from build123d import *

# Parameters (mm, degrees)
SKETCH1_W           = 10
SKETCH1_H           = 90
BOSS_EXTRUDE1_DEPTH = 10
CUT_EXTRUDE1_DEPTH  = 91
CUT_EXTRUDE2_DEPTH  = 91
CUT_EXTRUDE3_DEPTH  = 91
CUT_EXTRUDE4_DEPTH  = 91
FILLET1_R           = 0.2


with BuildPart() as part:
    # Sketch1 → Boss-Extrude1 (new body)
    with BuildSketch(Plane(origin=(0, 5, 0), x_dir=(1, 0, 0), z_dir=(0, 1, 0))):
        Rectangle(SKETCH1_W, SKETCH1_H)
    extrude(amount=-BOSS_EXTRUDE1_DEPTH)

    # Sketch2 → Cut-Extrude1 (cut, through all)
    with BuildSketch(Plane.XY.offset(45)):
        with BuildLine():
            Line((5, 1.5), (4, 1.5))
            Line((4, 1.5), (4, 2.759344808))
            ThreePointArc((4, 2.759344808), (3.870199868, 2.946619949), (3.649280215, 2.890811711))
            Line((3.649280215, 2.890811711), (2, 1))
            Line((2, 1), (2, -1))
            Line((2, -1), (3.649280215, -2.890811711))
            ThreePointArc((3.649280215, -2.890811711), (3.870199868, -2.946619949), (4, -2.759344808))
            Line((4, -2.759344808), (4, -1.5))
            Line((4, -1.5), (5, -1.5))
            Line((5, -1.5), (5, 1.5))
        make_face()
    extrude(amount=-CUT_EXTRUDE1_DEPTH, mode=Mode.SUBTRACT)

    # Sketch3 → Cut-Extrude2 (cut, through all)
    with BuildSketch(Plane.XY.offset(45)):
        with BuildLine():
            Line((1.5, -5), (1.5, -4))
            Line((1.5, -4), (2.759344808, -4))
            ThreePointArc((2.759344808, -4), (2.946619949, -3.870199868), (2.890811711, -3.649280215))
            Line((2.890811711, -3.649280215), (1, -2))
            Line((1, -2), (-1, -2))
            Line((-1, -2), (-2.890811711, -3.649280215))
            ThreePointArc((-2.890811711, -3.649280215), (-2.946619949, -3.870199868), (-2.759344808, -4))
            Line((-2.759344808, -4), (-1.5, -4))
            Line((-1.5, -4), (-1.5, -5))
            Line((-1.5, -5), (1.5, -5))
        make_face()
    extrude(amount=-CUT_EXTRUDE2_DEPTH, mode=Mode.SUBTRACT)

    # Sketch4 → Cut-Extrude3 (cut, through all)
    with BuildSketch(Plane.XY.offset(45)):
        with BuildLine():
            Line((-5, -1.5), (-4, -1.5))
            Line((-4, -1.5), (-4, -2.759344808))
            ThreePointArc((-4, -2.759344808), (-3.870199868, -2.946619949), (-3.649280215, -2.890811711))
            Line((-3.649280215, -2.890811711), (-2, -1))
            Line((-2, -1), (-2, 1))
            Line((-2, 1), (-3.649280215, 2.890811711))
            ThreePointArc((-3.649280215, 2.890811711), (-3.870199868, 2.946619949), (-4, 2.759344808))
            Line((-4, 2.759344808), (-4, 1.5))
            Line((-4, 1.5), (-5, 1.5))
            Line((-5, 1.5), (-5, -1.5))
        make_face()
    extrude(amount=-CUT_EXTRUDE3_DEPTH, mode=Mode.SUBTRACT)

    # Sketch5 → Cut-Extrude4 (cut, through all)
    with BuildSketch(Plane.XY.offset(45)):
        with BuildLine():
            Line((-1.5, 5), (-1.5, 4))
            Line((-1.5, 4), (-2.759344808, 4))
            ThreePointArc((-2.759344808, 4), (-2.946619949, 3.870199868), (-2.890811711, 3.649280215))
            Line((-2.890811711, 3.649280215), (-1, 2))
            Line((-1, 2), (1, 2))
            Line((1, 2), (2.890811711, 3.649280215))
            ThreePointArc((2.890811711, 3.649280215), (2.946619949, 3.870199868), (2.759344808, 4))
            Line((2.759344808, 4), (1.5, 4))
            Line((1.5, 4), (1.5, 5))
            Line((1.5, 5), (-1.5, 5))
        make_face()
    extrude(amount=-CUT_EXTRUDE4_DEPTH, mode=Mode.SUBTRACT)

    # Sketch6 → Cut-Revolve1 (revolve, cut)
    with BuildSketch(Plane(origin=(0, 0, 0), x_dir=(1, 0, 0), z_dir=(0, 1, 0))):
        Polygon((1.499999999, 37), (1.25, 36.849784845), (1.25, -36.849784845), (1.499999999, -37), (1.499999999, -45), (0, -45), (0, 45), (1.499999999, 45), align=None)
    revolve(axis=Axis((0, 0, -45), (0, 0, 1)), mode=Mode.SUBTRACT)

    # Fillet1
    fillet1_edges = [part.edges().sort_by_distance(p)[0] for p in [
        (-5, -5, 0),
        (-1.5, 5, 0),
        (1.5, 5, 0),
        (1.5, 4, 0),
        (1, 2, 0),
        (-1, 2, 0),
        (-1.5, 4, 0),
        (5, 1.5, 0),
        (5, -1.5, 0),
        (4, -1.5, 0),
        (2, -1, 0),
        (2, 1, 0),
        (4, 1.5, 0),
        (5, -5, 0),
        (-5, 5, 0),
        (5, 5, 0),
        (1.5, -5, 0),
        (-1.5, -5, 0),
        (-1.5, -4, 0),
        (-1, -2, 0),
        (1, -2, 0),
        (1.5, -4, 0),
        (-5, -1.5, 0),
        (-5, 1.5, 0),
        (-4, 1.5, 0),
        (-2, 1, 0),
        (-2, -1, 0),
        (-4, -1.5, 0),
    ]]
    fillet(fillet1_edges, radius=FILLET1_R)


solid = part.part
Model file for the job. Use its own axes, mm. A direction names the side the tool comes from. Give positions to 0.01 mm unless a question says otherwise; leave off trailing zeros. Order: outer loops, then holes, each group sorted by start corner. A loop starts at its lowest first (then second) coordinate and runs counter-clockwise, first axis right, second up. Notation, with made-up numbers: (-1, 43) - (19, 43) arc R25 ccw to (19, 63) - close; hole circle Ø5 at (29, -21.5). An arc over 180 degrees is marked (long way). Write item = value, one per line. Start each with the question number.
1. Probe line 1 along Y through (x, z) = (-3.75, 20); line 2 along X through (y, z) = (4.75, 26.5); line 3 along Y through (x, z) = (-1.75, -39). List the from-to ranges inside material, lowest first.
2. Drop flat-ended pins along their axis: P1, Ø0.9, axis at y = 0.5, z = -7.5, coming from the -X side; P2, Ø1.5, axis at x = 0.5, z = -6, coming from the +Y side; P3, Ø0.9, axis at x = 0.5, z = 19, coming from the -Y side. Give the stop position or say it passes through.
3. Cut at A-A, the plane y = 0. List the corners of the cut face in (x, z).
4. Which spindle directions (+Z, -Z, +X, -X, +Y, -Y) get a long thin tool onto all of the face, cutting with end or side? Do faces 5 (the flat face through (2.84, -1.96, 0.63)), 6 (the flat face through (0, 2, 1)), 7 (the flat face through (0, -2, 1)). Say none if no direction does.
5. Two-plate mould, pull along Y, no slides. Class faces 1 (the flat face through (-3, 5, -1)), 2 (the flat face through (3, -5, -1)), 3 (the flat face through (-1.2, 1.2, -45)), 4 (the flat face through (-2.86, -1.986, 0.63)): pulls with the +Y half, pulls with the -Y half, needs draft (parallel to the pull), parting line crosses it, or undercut.
Taken from the geometry:
q1.line_1 = -5 to -2.95, 2.95 to 5
q1.line_2 = -5 to -1.5, 1.5 to 5
q1.line_3 = -5 to -4, -2.65 to 2.65, 4 to 5
q2.P1 = -2
q2.P2 = 2.22
q2.P3 = -2
q3.outline = (-2, -45) - (-1.5, -45) - (-1.5, -37) - (-1.25, -36.85) - (-1.25, 36.85) - (-1.5, 37) - (-1.5, 45) - (-2, 45) - close; (1.25, -36.85) - (1.5, -37) - (1.5, -45) - (2, -45) - (2, 45) - (1.5, 45) - (1.5, 37) - (1.25, 36.85) - close
q4.face_5 = +Z, -Z
q4.face_6 = +Z, -Z, +Y
q4.face_7 = +Z, -Z, -Y
q5.face_1 = pulls with the +Y half
q5.face_2 = pulls with the -Y half
q5.face_3 = needs draft
q5.face_4 = undercut
